Model file for the job. Use its own axes, mm. A direction names the side the tool comes from. Give positions to 0.01 mm unless a question says otherwise; leave off trailing zeros. Loops run counter-clockwise (first coordinate to the right, second up) from the corner with the lowest first, then second, coordinate; pieces in that order, holes last. Notation, with made-up numbers: M 28,17 L 80,17 A30 ccw 80,43 Z; hole C 77,49 d7. An arc over 180 degrees is marked long. Answer in a Markdown table with one row per item.
```python
from build123d import *

# Parameters (mm, degrees)
F3_DEPTH = 78.001


with BuildPart() as f1:
    # F0 (on Front) → F1 (revolve)
    with BuildSketch(Plane.XZ):
        with BuildLine():
            Line((-27, 10), (41, 10))
            Line((41, 10), (41, 19))
            Line((41, 19), (40, 19))
            ThreePointArc((40, 19), (37.8786796564, 19.8786796564), (37, 22))
            Line((37, 22), (37, 45))
            Line((37, 45), (33, 45))
            Line((33, 45), (29.3465183566, 33.05))
            Line((29.3465183566, 33.05), (23.6534816434, 33.05))
            Line((23.6534816434, 33.05), (20, 45))
            Line((20, 45), (17, 45))
            Line((17, 45), (13.3465183566, 33.05))
            Line((13.3465183566, 33.05), (7.6534816434, 33.05))
            Line((7.6534816434, 33.05), (4, 45))
            Line((4, 45), (0, 45))
            Line((0, 45), (0, 70))
            Line((0, 70), (-4, 70))
            Line((-4, 70), (-7.6534816434, 58.05))
            Line((-7.6534816434, 58.05), (-13.3465183566, 58.05))
            Line((-13.3465183566, 58.05), (-17, 70))
            Line((-17, 70), (-20, 70))
            Line((-20, 70), (-23.6534816434, 58.05))
            Line((-23.6534816434, 58.05), (-29.3465183566, 58.05))
            Line((-29.3465183566, 58.05), (-33, 70))
            Line((-33, 70), (-37, 70))
            Line((-37, 70), (-37, 35))
            Line((-37, 35), (-32, 35))
            ThreePointArc((-32, 35), (-28.4644660941, 33.5355339059), (-27, 30))
            Line((-27, 30), (-27, 10))
        make_face()
    revolve(axis=Axis((1.6295525322, 0, 0), (1, 0, 0)))

    # F2 (on face) → F3 (cut, through all)
    with BuildSketch(Plane.YZ.offset(41)):
        with BuildLine():
            ThreePointArc((9.7979589711, 2), (-10, 0), (9.7979589711, -2))
            ThreePointArc((9.7979589711, -2), (9.9493615301, -1.0050896201), (10, 0))
            ThreePointArc((10, 0), (9.9493615301, 1.0050896201), (9.7979589711, 2))
        make_face()
        with BuildLine():
            ThreePointArc((10, 0), (9.9493615301, -1.0050896201), (9.7979589711, -2))
            Line((9.7979589711, -2), (12.2, -2))
            Line((12.2, -2), (12.2, 2))
            Line((12.2, 2), (9.7979589711, 2))
            ThreePointArc((9.7979589711, 2), (9.9493615301, 1.0050896201), (10, 0))
        make_face()
    extrude(amount=-F3_DEPTH, mode=Mode.SUBTRACT)


solid = f1.part
```
(1) Saw through at A-A, the plane x = 25.5. Give the cut face in (y, z), and give its area (3 significant figures).
Established:
| item | result |
|---|---|
| outline | C 0,0 d66.1; hole M 9.8,-2 L 12.2,-2 L 12.2,2 L 9.8,2 A10 ccw long Z |
| area | 3,110 mm2 |
(2) Flat gauge pins, fed straight in: P1, Ø3, axis at x = -2, z = -18.5, coming from the +Y side; P2, Ø1, axis at x = -28.5, z = -37.5, coming from the +Y side; P3, Ø2.5, axis at x = -0.5, y = 10.5, coming from the +Z side. Where does each tip first touch, or does it go through?
Established:
| item | result |
|---|---|
| P1 | stops at y = 67.9 |
| P2 | stops at y = 44.73 |
| P3 | stops at z = 69.39 |
(3) Mould opens along Z. For faces 4 (the cylindrical face through (-26.54, -17.44, 55.37)), 5 (the flat face through (41, 8, -8)), 6 (the cylindrical face through (-34, 21, -28)), 7 (the flat face through (7, 12.2, 0)) say: pulls with the +Z half, pulls with the -Z half, needs draft (parallel to the pull), parting line crosses it, or undercut.
Established:
| item | result |
|---|---|
| face 4 | parting line crosses it |
| face 5 | needs draft |
| face 6 | undercut |
| face 7 | undercut |
(4) Which spindle directions (+Z, -Z, +X, -X, +Y, -Y) get a long thin tool onto all of the face, cutting with end or side? Do faces 1 (the cylindrical face through (-2.028, 42.594, -55.55)), 2 (the conical face through (13.524, 20.463, -26.688)), 3 (the cylindrical face through (18.479, 39.923, 20.765)). Say none if no direction does.
Established:
| item | result |
|---|---|
| face 1 | +X, -X |
| face 2 | none |
| face 3 | +X |
(5) Wall check: L1, parallel to X at y = -12, z = -62; L2, parallel to Z at x = -35, y = 0; L3, parallel to Y at x = -10.5, z = 0. Give the ranges that are in metal, low to high.
Established:
| item | result |
|---|---|
| L1 | x = -37 to -30.91, -22.09 to -14.91, -6.09 to 0 |
| L2 | z = -70 to -35, 35 to 70 |
| L3 | y = -58.05 to -10, 12.2 to 58.05 |
